Print and shaded views of the part. All mm, measured from the part's lowest x, y and z. A direction names the side the tool comes from. Round coordinates to 2 decimals unless told otherwise and drop trailing zeros. Loops run counter-clockwise (first coordinate to the right, second up) from the corner with the lowest first, then second, coordinate; pieces in that order, holes last. Notation, with made-up numbers: (24, 74) -> (53, 74) arc R28 cw to (53, 95) -> close; hole circle Ø4 at (3.25, 20). An arc over 180 degrees is marked (long way). Answer as CSV lines item,"result".
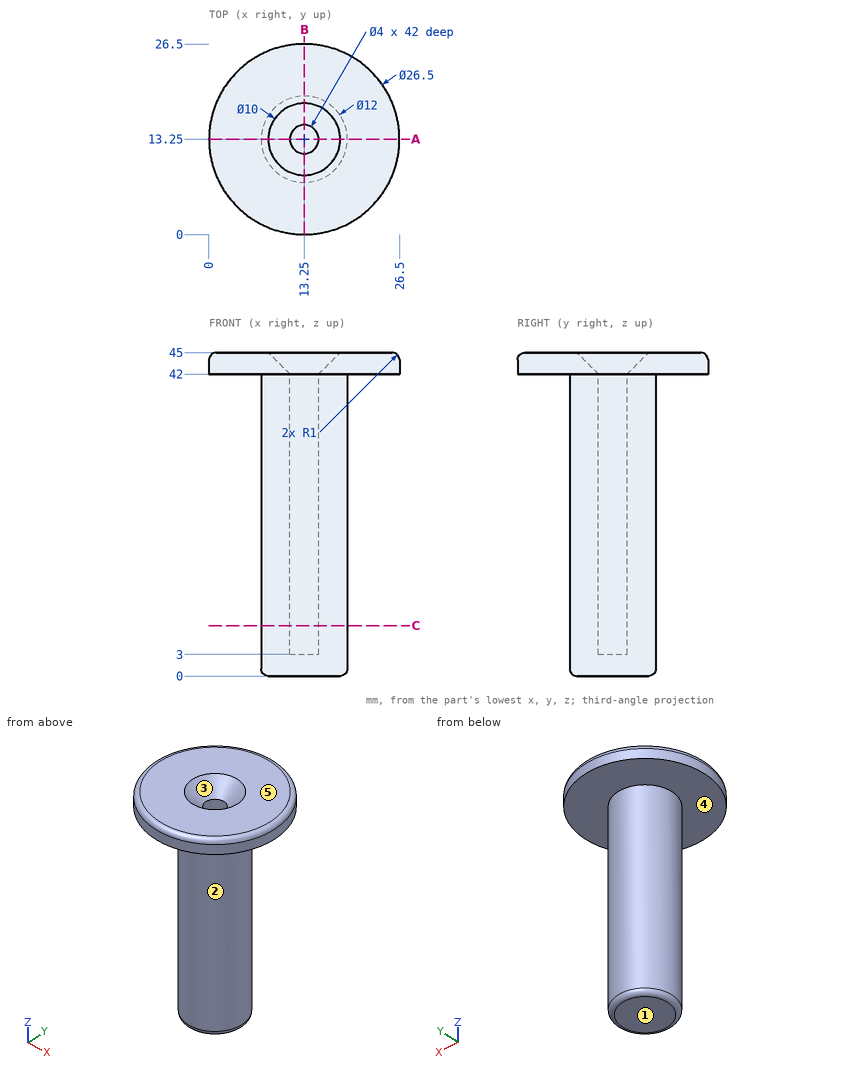
Q1. Tool access for the marked faces 4 and 5: list every direction of +Z, -Z, +X, -X, +Y, -Y with a clear straight run to the whole face (end or side of a thin tool).
Results:
face 4,"-Z"
face 5,"+Z, +X, -X, +Y, -Y"
Q2. Drop flat-ended pins along their axis: pin 1 Ø3 at (x, y) = (11.5, 16.5) entering from -Z; pin 2 Ø6 at (x, z) = (11, 33.5) entering from +Y; pin 3 Ø5 at (x, y) = (13, 23) entering from -Z; pin 4 Ø4.5 at (x, y) = (14, 13.5) entering from +Z. Give the stop position or say it passes through.
Results:
pin 1,"z = 0"
pin 2,"y = 19.25"
pin 3,"z = 42"
pin 4,"z = 43.04"
Q3. Probe L1, parallel to Y at x = 13.25, z = 29.5; L2, parallel to Z at x = 22.5, y = 18. List the from-to ranges inside material, lowest first. Write a range as [from, to].
Results:
L1,"[7.25, 11.25], [15.25, 19.25]"
L2,"[42, 45]"
Q4. Two-plate mould, pull along Y, no slides. Class the marked faces 1, 2 and 3: pulls with the +Y half, pulls with the -Y half, needs draft (parallel to the pull), parting line crosses it, or undercut.
Results:
face 1,"needs draft"
face 2,"parting line crosses it"
face 3,"undercut"
Q5. Slice it at A-A, the plane y = 13.25. Give the cut face in (x, z).
Results:
outline,"(0, 42) -> (7.25, 42) -> (7.25, 1) arc R1 ccw to (8.25, 0) -> (18.25, 0) arc R1 ccw to (19.25, 1) -> (19.25, 42) -> (26.5, 42) -> (26.5, 44) arc R1 ccw to (25.5, 45) -> (18.25, 45) -> (15.25, 42) -> (15.25, 3) -> (11.25, 3) -> (11.25, 42) -> (8.25, 45) -> (1, 45) arc R1 ccw to (0, 44) -> close"
Q6. Slice it at C-C, the plane z = 7. Give the cut face in (x, y).
Results:
outline,"circle Ø12 at (13.25, 13.25); hole circle Ø4 at (13.25, 13.25)"
